Input: part model. Units: mm. Frame: model coordinates. A direction names the side the tool comes from. Give positions to 0.01 mm unless a question says otherwise; leave off trailing zeros. Loops run counter-clockwise (first coordinate to the right, second up) from the corner with the lowest first, then second, coordinate; pieces in that order, holes last. Notation, with made-up numbers: M -27,-22.75 L -14,-22.75 A27 cw -14,12.25 Z; hole C 16,-10 d4. An arc over 180 degrees is marked long. One line per item, written item: value. Start each with the question number.
(1) Pin query (flat end, axial travel): P1, Ø2.5, axis at x = -41.25, z = -45.46, coming from the -Y side; P2, Ø6.5, axis at x = 84.5, z = 16.5, coming from the +Y side; P3, Ø6, axis at x = 36, y = 20, coming from the -Z side; P4, Ø6.5, axis at x = 85.7, z = 16.26, coming from the +Y side. Return the tip coordinate at first contact, or that it passes through.
(2) Pull-direction query (Z, two-part tool) for faces 1 (the flat face through (21, 15, 36.75)), 2 (the flat face through (97.658, 17, -13)), 3 (the cylindrical face through (89.666, 4.754, 15.736)); classes: released by +Z, released by -Z, zero draft, split by the parting line, or undercut.
(3) Access query for faces 4 (the flat face through (21, 5, -14)), 5 (the flat face through (22, 2, -53.37)), 6 (the flat face through (86.1, 4.5, -43.7)). Directions: +Z, -Z, +X, -X, +Y, -Y. A direction counts if a zero-diameter tool reaches every point of the face in a straight line with its end or side. Return the directions, or none.
(4) Section A-A on z = -3. Output: boundary loops of the cut face in (x, y).
(5) Section C-C on x = 8. Output: boundary loops of the cut face in (y, z).
(6) Section B-B on y = 25.75. Output: boundary loops of the cut face in (x, z), plus the area to 3 significant figures.
(7) Ray query, line 1 along X through (y, z) = (16.75, -23); line 2 along Y through (x, z) = (2.5, -10); line 3 along Z through (x, y) = (-30.5, 14.75). Return the intervals inside material, ascending. Write a range as from..to.
```python
from build123d import *

# Parameters (mm, degrees)
SKETCH1_W                                            = 151.33
SKETCH1_H                                            = 80.12
BOSS_EXTRUDE1_DEPTH                                  = 5
SKETCH3_W                                            = 10
SKETCH3_H                                            = 90.12
SKETCH3_W_2                                          = 151.33
SKETCH3_H_2                                          = 10
BOSS_EXTRUDE2_DEPTH                                  = 30
CBORE_FOR_M2_5_HEXAGON_HEAD_BOLTS_FULL_T_D           = 2.9
CBORE_FOR_M2_5_HEXAGON_HEAD_BOLTS_FULL_T_DEPTH       = 20
CBORE_FOR_M2_5_HEXAGON_HEAD_BOLTS_FULL_T_CBORE_D     = 8
CBORE_FOR_M2_5_HEXAGON_HEAD_BOLTS_FULL_T_CBORE_DEPTH = 0.5
CBORE_FOR_M2_5_HEXAGON_HEAD_BOLTS_FULL_T_TIP         = 0.871247898


with BuildPart() as part:
    # Sketch1 → Boss-Extrude1 (new body)
    with BuildSketch(Plane(origin=(0, 0, 0), x_dir=(1, 0, 0), z_dir=(0, 1, 0))):
        with Locations((21.993286604, 13.310186916)):
            Rectangle(SKETCH1_W, SKETCH1_H)
    extrude(amount=BOSS_EXTRUDE1_DEPTH)

    # Sketch3 → Boss-Extrude2 (add)
    with BuildSketch(Plane(origin=(0, 0, 0), x_dir=(1, 0, 0), z_dir=(0, 1, 0))):
        with Locations((-58.671713396, 8.310186916)):
            Rectangle(SKETCH3_W, SKETCH3_H)
        with Locations((21.993286604, -31.749813084)):
            Rectangle(SKETCH3_W_2, SKETCH3_H_2)
        with Locations((102.658286604, 8.310186916)):
            Rectangle(SKETCH3_W, SKETCH3_H)
    extrude(amount=BOSS_EXTRUDE2_DEPTH)

    # CBORE for M2.5 Hexagon head bolts-Full thread-grades AB1
    with Locations(Plane(origin=(85.700408956, 5, 16.256611899), x_dir=(0, 0, 1), z_dir=(0, 1, 0))):
        with Locations((0, 0), (0.080180531, -126.947449906), (-61.719848362, -126.947449906), (-61.719848362, 0.369580631)):
            CounterBoreHole(CBORE_FOR_M2_5_HEXAGON_HEAD_BOLTS_FULL_T_D / 2, CBORE_FOR_M2_5_HEXAGON_HEAD_BOLTS_FULL_T_CBORE_D / 2, CBORE_FOR_M2_5_HEXAGON_HEAD_BOLTS_FULL_T_CBORE_DEPTH, depth=CBORE_FOR_M2_5_HEXAGON_HEAD_BOLTS_FULL_T_DEPTH)
            with Locations((0, 0, -(CBORE_FOR_M2_5_HEXAGON_HEAD_BOLTS_FULL_T_DEPTH + CBORE_FOR_M2_5_HEXAGON_HEAD_BOLTS_FULL_T_TIP / 2))):  # 118° drill point
                Cone(0, CBORE_FOR_M2_5_HEXAGON_HEAD_BOLTS_FULL_T_D / 2, CBORE_FOR_M2_5_HEXAGON_HEAD_BOLTS_FULL_T_TIP, mode=Mode.SUBTRACT)


solid = part.part
```
Output values:
1. P1: passes through
1. P2: stops at y = 5
1. P3: stops at z = 26.75
1. P4: stops at y = 4.5
2. face 1: released by +Z
2. face 2: zero draft
2. face 3: undercut
3. face 4: -Z, +Y
3. face 5: -Z, +X, -X, +Y, -Y
3. face 6: +Y
4. outline: M -63.67,0 L 107.66,0 L 107.66,30 L 97.66,30 L 97.66,5 L -53.67,5 L -53.67,30 L -63.67,30 Z
5. outline: M 0,-53.37 L 5,-53.37 L 5,26.75 L 30,26.75 L 30,36.75 L 0,36.75 Z
6. outline: M -63.67,-53.37 L -53.67,-53.37 L -53.67,26.75 L 97.66,26.75 L 97.66,-53.37 L 107.66,-53.37 L 107.66,36.75 L -63.67,36.75 Z
6. area: 3,320 mm²
7. line 1: x = -63.67..-53.67, 97.66..107.66
7. line 2: y = 0..5
7. line 3: z = 26.75..36.75
